```python
from build123d import *

# Parameters (mm, degrees)
F0_R     = 20
F1_DEPTH = 100
F2_SIZE  = 5
F4_DEPTH = 100.001


with BuildPart() as f1:
    # F0 (on Top) → F1 (new body)
    with BuildSketch(Plane.XY):
        Circle(F0_R)
    extrude(amount=F1_DEPTH)

    # F2
    f2_edges = [f1.edges().sort_by_distance(p)[0] for p in [
        (-20, 0, 100),
    ]]
    chamfer(f2_edges, length=F2_SIZE)

    # F3 (on face) → F4 (cut, through all)
    with BuildSketch(Plane.XY.offset(100)):
        Polygon((0.03937, -5.773368), (5.019569, -2.852589), (4.980199, 2.920779), (-0.03937, 5.773368), (-5.019569, 2.852589), (-4.980199, -2.920779), align=None)
    extrude(amount=-F4_DEPTH, mode=Mode.SUBTRACT)


solid = f1.part
```
The model under review builds one solid part; all positions refer to its coordinate system, in mm. A direction names the side the tool comes from. Give positions to 0.01 mm unless a question says otherwise; leave off trailing zeros. Write each loop counter-clockwise with the first axis right and the second up, starting at its lowest first coordinate (ties: lowest second). Pieces come first, ordered by that corner, then holes.
(1) To check wall thickness, follow L1, parallel to X at y = -2, z = 15; L2, parallel to Y at x = 2, z = 72; L3, parallel to Y at x = 11, z = 51. State the ranges of each line that lie inside material, in increasing order.
(2) The part is to be moulded in two halves that separate along Y. For faces 3 (the flat face through (2.506, 4.327, 50.7)), 4 (the conical face through (14.539, 4.579, 99.757)), 5 (the flat face through (2.495, -4.333, 50.7)), 6 (the flat face through (4, -4, 0)), say which applies: released by +Y, released by -Y, zero draft, split by the parting line, or undercut.
(3) For P1, Ø1.5, axis at y = 4.5, z = 68.5, coming from the -X side; P2, Ø2, axis at x = 13.5, z = 54, coming from the -Y side; P3, Ø12, axis at x = 4.5, z = 43, coming from the +Y side, all flat-tipped, find the tip position at first contact; note any pin that passes through.
(4) Consider section B-B, the plane y = 0. Give the boundary of the cut face in (x, z), and give its area (3 significant figures).
(5) Consider section A-A, the plane z = 9. Give the boundary of the cut face in (x, y), and give its area (3 significant figures).
(6) Tool access review of faces 1 (the flat face through (6, 0, 100)), 2 (the flat face through (-2.506, -4.327, 50.7)): name each direction out of +Z, -Z, +X, -X, +Y, -Y from which nothing blocks a thin tool from reaching the whole face with its end or side.
Returned:
1. L1: x = -19.9 to -4.99, 5.01 to 19.9
1. L2: y = -19.9 to -4.62, 4.61 to 19.9
1. L3: y = -16.7 to 16.7
2. face 3: undercut
2. face 4: split by the parting line
2. face 5: undercut
2. face 6: zero draft
3. P1: stops at x = -19.65
3. P2: stops at y = -15.61
3. P3: stops at y = 20
4. outline: (-20, 0) - (-5, 0) - (-5, 100) - (-15, 100) - (-20, 95) - close; (5, 0) - (20, 0) - (20, 95) - (15, 100) - (5, 100) - close
4. area: 2,970 mm2
5. outline: circle Ø40 at (0, 0); hole (-5.02, 2.85) - (-4.98, -2.92) - (0.04, -5.77) - (5.02, -2.85) - (4.98, 2.92) - (-0.04, 5.77) - close
5. area: 1,170 mm2
6. face 1: +Z, +X, -X, +Y, -Y
6. face 2: +Z, -Z
